The listing builds one solid part. Answer for the finished solid, in the listing's coordinates (mm). Face numbers are marked on the shaded views. Coordinates: 2 decimals unless noted, no trailing zeros. Write each loop counter-clockwise with the first axis right and the second up, starting at its lowest first coordinate (ties: lowest second). Pieces come first, ordered by that corner, then holes.
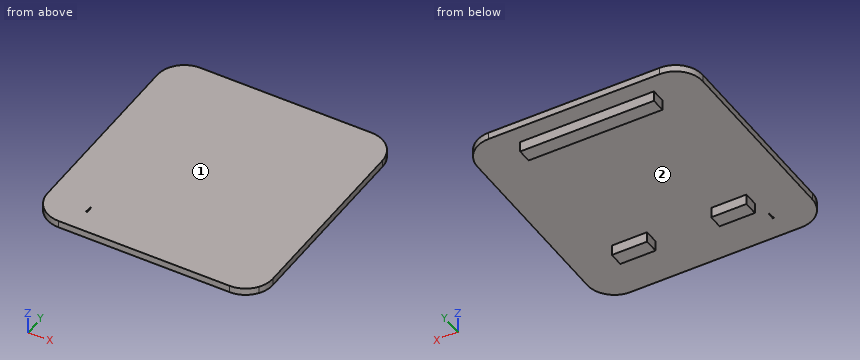
from build123d import *

# Parameters (mm, degrees)
F1_DEPTH = 2
F2_DEPTH = 2
F4_W     = 38
F4_H     = 4
F4_W_2   = 10
F5_DEPTH = 3


# Not quite as in the source:
# - a feature names something its author has since deleted; it is built from what else it names


with BuildPart() as f1:
    # F0 (on Top) → F1 (new body)
    with BuildSketch(Plane.XY):
        with BuildLine():
            Line((24.3022678875, 34), (-24.3022678875, 34))
            ThreePointArc((-24.3022678875, 34), (-29.745386464, 31.745386464), (-32, 26.3022678875))
            Line((-32, 26.3022678875), (-32, 15.1276998222))
            Line((-32, 15.1276998222), (-30.5, 15.1276998222))
            Line((-30.5, 15.1276998222), (-30.5, 21.3020170704))
            Line((-30.5, 21.3020170704), (30.5, 21.3020170704))
            Line((30.5, 21.3020170704), (30.5, 14.2477769405))
            Line((30.5, 14.2477769405), (32, 14.2477769405))
            Line((32, 14.2477769405), (32, 26.3022678875))
            ThreePointArc((32, 26.3022678875), (29.745386464, 31.745386464), (24.3022678875, 34))
        make_face()
        with BuildLine():
            Line((-30.5, 15.1276998222), (-32, 15.1276998222))
            Line((-32, 15.1276998222), (-32, -26.3022678875))
            ThreePointArc((-32, -26.3022678875), (-29.745386464, -31.745386464), (-24.3022678875, -34))
            Line((-24.3022678875, -34), (0, -34))
            Line((0, -34), (24.3022678875, -34))
            ThreePointArc((24.3022678875, -34), (27.9138443036, -33.100178998), (30.6810753302, -30.6110838832))
            ThreePointArc((30.6810753302, -30.6110838832), (31.6628871063, -28.555346757), (32, -26.3022678875))
            Line((32, -26.3022678875), (32, 14.2477769405))
            Line((32, 14.2477769405), (30.5, 14.2477769405))
            Line((30.5, 14.2477769405), (30.5, -14.6979829296))
            Line((30.5, -14.6979829296), (-30.5, -14.6979829296))
            Line((-30.5, -14.6979829296), (-30.5, 15.1276998222))
        make_face()
        with BuildLine():
            ThreePointArc((-20.3994758379, -27.4899639189), (-30.2031719041, -25.7844938681), (-20.255592559, -25.5261339915))
            Line((-20.255592559, -25.5261339915), (-20, -25.5261339915))
            Line((-20, -25.5261339915), (-20, -27.4899639189))
            Line((-20, -27.4899639189), (-20.3994758379, -27.4899639189))
        make_face(mode=Mode.SUBTRACT)
        with BuildLine():
            ThreePointArc((20.2726339823, -25.4029799253), (25.5910239568, -21.1638916046), (30.2165381279, -26.1498479185))
            ThreePointArc((30.2165381279, -26.1498479185), (25.7296627026, -31.1234485429), (20.3218568596, -27.1706786007))
            ThreePointArc((20.3218568596, -27.1706786007), (20.2184754644, -26.2890226707), (20.2726339823, -25.4029799253))
        make_face(mode=Mode.SUBTRACT)
        Polygon((-30.5, 21.3020170704), (-30.5, 15.1276998222), (-30.5, -14.6979829296), (30.5, -14.6979829296), (30.5, 14.2477769405), (30.5, 21.3020170704), align=None)
    extrude(amount=F1_DEPTH)

    # F0 (on Top) → F2 (join)
    with BuildSketch(Plane.XY):
        with BuildLine():
            ThreePointArc((-20.3994758379, -27.4899639189), (-20.2624836545, -26.8261202565), (-20.2165381279, -26.1498479185))
            ThreePointArc((-20.2165381279, -26.1498479185), (-20.2263112871, -25.8373801956), (-20.255592559, -25.5261339915))
            ThreePointArc((-20.255592559, -25.5261339915), (-30.2031719041, -25.7844938681), (-20.3994758379, -27.4899639189))
        make_face()
        with BuildLine():
            ThreePointArc((20.3218568596, -27.1706786007), (25.7296627026, -31.1234485429), (30.2165381279, -26.1498479185))
            ThreePointArc((30.2165381279, -26.1498479185), (25.5910239568, -21.1638916046), (20.2726339823, -25.4029799253))
            ThreePointArc((20.2726339823, -25.4029799253), (20.2184754644, -26.2890226707), (20.3218568596, -27.1706786007))
        make_face()
    extrude(amount=F2_DEPTH)

    # F4 (on face) → F5 (join)
    with BuildSketch(Plane.XY):
        with Locations((-0.7767596692, 27.0571730584)):
            Rectangle(F4_W, F4_H)
        with Locations((14.1091264039, -18.375430584)):
            Rectangle(F4_W_2, F4_H)
        with Locations((-14.1091264039, -18.375430584)):
            Rectangle(F4_W_2, F4_H)
    extrude(amount=-F5_DEPTH)


solid = f1.part
Q1. The part is cut by section A-A, the plane z = -0.9. Write down the section's boundary in (x, y).
Answers below:
outline: (-19.78, 25.06) - (18.22, 25.06) - (18.22, 29.06) - (-19.78, 29.06) - close; (-19.11, -20.38) - (-9.11, -20.38) - (-9.11, -16.38) - (-19.11, -16.38) - close; (9.11, -20.38) - (19.11, -20.38) - (19.11, -16.38) - (9.11, -16.38) - close
Q2. The part is cut by section D-D, the plane x = -16. Write down the section's boundary in (y, z), then the cut area to 3 significant figures.
Answers below:
outline: (-34, 0) - (-20.38, 0) - (-20.38, -3) - (-16.38, -3) - (-16.38, 0) - (25.06, 0) - (25.06, -3) - (29.06, -3) - (29.06, 0) - (34, 0) - (34, 2) - (-34, 2) - close
area: 160 mm2
Q3. Given pin 1 (6 mm diameter, centred on x = -2.5, y = -25.5, fed in from -Z); pin 2 (2.5 mm diameter, centred on x = -14, z = -2, fed in from -Y); pin 3 (0.9 mm diameter, centred on x = -6, z = -2, fed in from +Y), each flat-ended and moving along its own axis, determine where each tip first touches the part or whether it passes through.
Answers below:
pin 1: stops at z = 0
pin 2: stops at y = -20.38
pin 3: stops at y = 29.06
Q4. The part is cut by section C-C, the plane y = -0.5. Write down the section's boundary in (x, z).
Answers below:
outline: (-32, 0) - (32, 0) - (32, 2) - (-32, 2) - close
Q5. Determine the mould class of the marked faces 1 and 2 for opening direction Y: released by +Y, released by -Y, zero draft, split by the parting line, or undercut.
Answers below:
face 1: zero draft
face 2: undercut
Q6. Find the intervals of material crossed by probe 1 along X at (y, z) = (-19.5, -1.25); probe 2 along Y at (x, z) = (17.5, -0.5); probe 3 along Z at (x, y) = (29.5, -12), in increasing order.
Answers below:
probe 1: x = -19.11 to -9.11, 9.11 to 19.11
probe 2: y = -20.38 to -16.38, 25.06 to 29.06
probe 3: z = 0 to 2
Q7. The part is cut by section B-B, the plane x = -7.5. Write down the section's boundary in (y, z), then the cut area to 3 significant figures.
Answers below:
outline: (-34, 0) - (25.06, 0) - (25.06, -3) - (29.06, -3) - (29.06, 0) - (34, 0) - (34, 2) - (-34, 2) - close
area: 148 mm2
